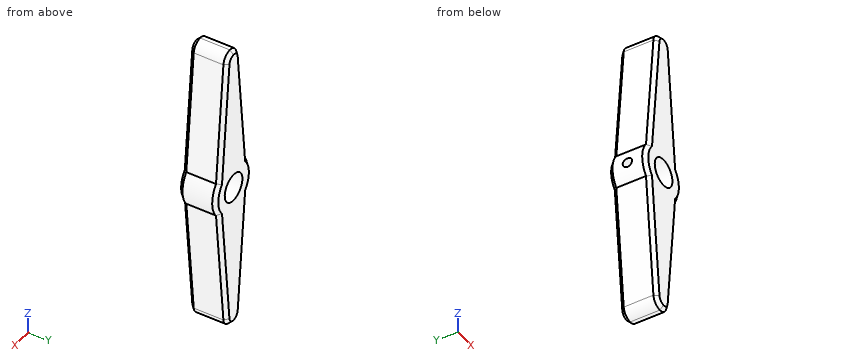
from build123d import *

# Parameters (mm, degrees)
SKETCH1_R               = 9.525
BOSS_EXTRUDE1_DEPTH     = 6.35
BOSS_EXTRUDE2_DEPTH     = 6.35
FILLET1_R               = 3.49359
FILLET1_OF_MIRROR2_R    = 3.49359
CHAMFER1_SIZE           = 1.27
CUT_EXTRUDE1_DEPTH      = 53.073871807
CUT_EXTRUDE1_DEPTH_BACK = 53.073871807
SKETCH1_3_R             = 4.7625
SKETCH3_R               = 1.5875
CUT_EXTRUDE2_DEPTH      = 53.073871807


with BuildPart() as part:
    # Sketch1 → Boss-Extrude1 (new, symmetric)
    with BuildSketch(Plane(origin=(0, 0, 0), x_dir=(1, 0, 0), z_dir=(0, 1, 0))):
        with Locations(Location((0, 0, 0), (0, 0, 270))):
            Circle(SKETCH1_R)
    extrude(amount=BOSS_EXTRUDE1_DEPTH, both=True)

    # Sketch2 → Boss-Extrude2 (add, symmetric)
    with BuildSketch(Plane(origin=(0, 0, 0), x_dir=(1, 0, 0), z_dir=(0, 1, 0))):
        Polygon((-8.040009509, 0), (8.040009509, 0), (3.175, 50.8), (-3.175, 50.8), align=None)
    boss_extrude2 = extrude(amount=BOSS_EXTRUDE2_DEPTH, both=True)

    # Fillet1
    fillet1_edges = [part.edges().sort_by_distance(p)[0] for p in [
        (-3.175, 0, -50.8),
        (3.175, 0, -50.8),
    ]]
    fillet(fillet1_edges, radius=FILLET1_R - 0.0001)  # a hair under: the kernel refuses the full size

    # Mirror2: Boss-Extrude2 across plane
    add(boss_extrude2.mirror(Plane.XY))

    # Fillet1 of Mirror2
    fillet1_of_mirror2_edges = [part.edges().sort_by_distance(p)[0] for p in [
        (-3.175, 0, 50.8),
        (3.175, 0, 50.8),
    ]]
    fillet(fillet1_of_mirror2_edges, radius=FILLET1_OF_MIRROR2_R - 0.0001)  # a hair under: the kernel refuses the full size

    # Chamfer1
    chamfer1_edges = [part.edges().sort_by_distance(p)[0] for p in [
        (5.476138131, -6.35, -26.771718685),
        (5.476138131, 6.35, -26.771718685),
        (-5.476138131, -6.35, -26.771718685),
        (-5.476138131, 6.35, -26.771718685),
        (0, -6.35, -50.8),
        (0, 6.35, -50.8),
        (9.525, -6.35, 0),
        (9.525, 6.35, 0),
        (5.476138131, 6.35, 26.771718685),
        (5.476138131, -6.35, 26.771718685),
        (-9.525, -6.35, 0),
        (-5.476138131, -6.35, 26.771718685),
        (-5.476138131, 6.35, 26.771718685),
        (0, 6.35, 50.8),
        (0, -6.35, 50.8),
        (-9.525, 6.35, 0),
    ]]
    chamfer(chamfer1_edges, length=CHAMFER1_SIZE)

    # Sketch1<3> → Cut-Extrude1 (cut, two sides: drawn at the far end of the back side and taken through both)
    with BuildSketch(Plane(origin=(0, 0, 0), x_dir=(1, 0, 0), z_dir=(0, 1, 0)).offset(-CUT_EXTRUDE1_DEPTH_BACK)):
        with Locations(Location((0, 0, 0), (0, 0, 270))):
            Circle(SKETCH1_3_R)
    extrude(amount=CUT_EXTRUDE1_DEPTH + CUT_EXTRUDE1_DEPTH_BACK, mode=Mode.SUBTRACT)

    # Sketch3 → Cut-Extrude2 (cut, through all)
    with BuildSketch(Plane(origin=(0, 0, 0), x_dir=(0, 0, -1), z_dir=(1, 0, 0))):
        Circle(SKETCH3_R)
    extrude(amount=-CUT_EXTRUDE2_DEPTH, mode=Mode.SUBTRACT)


solid = part.part
Here's how the part is built. I have some questions about the finished solid (model axes, mm). Round coordinates to 2 decimals unless told otherwise and drop trailing zeros. Write each loop counter-clockwise with the first axis right and the second up, starting at its lowest first coordinate (ties: lowest second). Pieces come first, ordered by that corner, then holes.
1. Suppose I cut it at D-D (z = 14). List the corners of the cut face in (x, y) for me.
2. Will these pins go through, and if not, where does the flat tip stop? pin 1 Ø4 at (x, y) = (4, -1) entering from +Z; pin 2 Ø1 at (y, z) = (3.5, -37.5) entering from +X; pin 3 Ø5 at (x, y) = (5.5, -0.5) entering from +Z.
3. Suppose I cut it at B-B (z = 0). State how many separate pieces and enclosed holes the cut face has, and give its area (3 significant figures).
4. I need wall thicknesses on L1, parallel to Y at x = -5.45, z = 0; L2, parallel to Z at x = 0, y = 1.75; L3, parallel to X at y = 2, z = 0 (1 decimal). Which ranges of each line are inside material? Lowest first, please.
5. Suppose I cut it at C-C (z = -36.5). List the corners of the cut face in (x, y) for me, and give its area (3 significant figures).
Answer sheet:
1. outline: (-6.7, -5.08) - (-5.42, -6.35) - (5.42, -6.35) - (6.7, -5.08) - (6.7, 5.08) - (5.42, 6.35) - (-5.42, 6.35) - (-6.7, 5.08) - close
2. pin 1: stops at z = 50.17
2. pin 2: stops at x = 4.5
2. pin 3: stops at z = 49.1
3. separate pieces: 3
3. enclosed holes: 0
3. area: 103 mm2
4. L1: y = -6.35 to -1.59, 1.59 to 6.35
4. L2: z = -50.8 to -4.76, 4.76 to 50.8
4. L3: x = -9.5 to -4.8, 4.8 to 9.5
5. outline: (-4.54, -5.08) - (-3.27, -6.35) - (3.27, -6.35) - (4.54, -5.08) - (4.54, 5.08) - (3.27, 6.35) - (-3.27, 6.35) - (-4.54, 5.08) - close
5. area: 112 mm2
